```python
from build123d import *

# Parameters (mm, degrees)
BOSS_EXTRUDE1_DEPTH = 546.1
SKETCH2_R           = 49.5046
SKETCH2_R_2         = 47.6885
BOSS_EXTRUDE2_DEPTH = 203.2
BOSS_EXTRUDE3_START = 101.6
SKETCH3_R           = 49.5046
SKETCH3_R_2         = 47.6885
BOSS_EXTRUDE3_DEPTH = 101.6
SKETCH4_R           = 3.175
CUT_EXTRUDE1_DEPTH  = 753.563552693
CIRPATTERN1_COUNT   = 4


with BuildPart() as part:
    # Sketch1 → Boss-Extrude1 (new body)
    with BuildSketch(Plane.XY):
        with BuildLine():
            Line((-49.5046, 0), (-47.6885, 0))
            ThreePointArc((-47.6885, 0), (0, -47.6885), (47.6885, 0))
            Line((47.6885, 0), (49.5046, 0))
            ThreePointArc((49.5046, 0), (0, -49.5046), (-49.5046, 0))
        make_face()
    extrude(amount=BOSS_EXTRUDE1_DEPTH)

    # Sketch2 → Boss-Extrude2 (add)
    with BuildSketch(Plane.XY.offset(546.1)):
        Circle(SKETCH2_R)
        Circle(SKETCH2_R_2, mode=Mode.SUBTRACT)
    extrude(amount=BOSS_EXTRUDE2_DEPTH)

    # Sketch3 → Boss-Extrude3 (add)
    with BuildSketch(Plane(origin=(0, 0, 0), x_dir=(-1, 0, 0), z_dir=(0, 0, -1)).offset(BOSS_EXTRUDE3_START)):
        Circle(SKETCH3_R)
        Circle(SKETCH3_R_2, mode=Mode.SUBTRACT)
    extrude(amount=-BOSS_EXTRUDE3_DEPTH)

    # Sketch4 → Cut-Extrude1 (cut, through all)
    with BuildSketch(Plane(origin=(0, 0, 0), x_dir=(1, 0, 0), z_dir=(0, 1, 0))):
        with Locations(Location((0, -698.5, 0), (0, 0, 270))):
            Circle(SKETCH4_R)
    cut_extrude1 = extrude(amount=-CUT_EXTRUDE1_DEPTH, mode=Mode.SUBTRACT)

    # CirPattern1: Cut-Extrude1 ×4 about axis
    cirpattern1_axis = Axis((0, 0, 546.1), (0, 0, -1))
    for i in range(1, CIRPATTERN1_COUNT):
        add(cut_extrude1.rotate(cirpattern1_axis, i * 360 / CIRPATTERN1_COUNT), mode=Mode.SUBTRACT)


solid = part.part
```
Model file for the job. Use its own axes, mm. Coordinates: 2 decimals unless noted, no trailing zeros. Order: outer loops, then holes, each group sorted by start corner. A loop starts at its lowest first (then second) coordinate and runs counter-clockwise, first axis right, second up. Notation, with made-up numbers: (-38.5, 57.5) - (12.5, 57.5) arc R14 ccw to (12.5, 80.5) - close; hole circle Ø11 at (62.5, 39). An arc over 180 degrees is marked (long way). Return JSON: item names as keys, results as strings. Group by question number.
1) Saw through at C-C, the plane y = 26. Write the cut outline in (x, z).
2) Saw through at B-B, the plane y = -36.5. Write the cut outline in (x, z), plus the area to 3 significant figures.
3) Saw through at A-A, the plane x = 40. Write the cut outline in (y, z), plus the area to 3 significant figures.
4) Probe line 1 (Y direction, x = -3, z = 511); line 2 (Z direction, x = 0, y = -48.2) (3 decimals); line 3 (X direction, y = -24, z = 492). List the from-to ranges inside material, lowest first. Write a range as from..to.
5) Mould opens along Z. For faces 1 (the flat face through (26, 41, -101.6)), 2 (the flat face through (0, 49, 546.1)), 3 (the flat face through (-26, 41, 749.3)) say: released by +Z, released by -Z, zero draft, split by the parting line, or undercut.
6) Flat gauge pins, fed straight in: P1, Ø12, axis at x = 14.5, z = 80, coming from the +Y side; P2, Ø1.5, axis at y = -16.5, z = 483, coming from the -X side; P3, Ø6, axis at x = -8, z = 636, coming from the +Y side; P4, Ø25, axis at x = -18, y = 16.5, coming from the +Z side. Where does each tip first touch, or does it go through?
7) Saw through at D-D, the plane z = 184. Write the cut outline in (x, y), plus the area to 3 significant figures.
Values found:
{
 "1": {"outline": "(-42.13, -101.6) - (-39.98, -101.6) - (-39.98, 0) - (-42.13, 0) - close; (-42.13, 546.1) - (-39.98, 546.1) - (-39.98, 749.3) - (-42.13, 749.3) - close; (39.98, -101.6) - (42.13, -101.6) - (42.13, 0) - (39.98, 0) - close; (39.98, 546.1) - (42.13, 546.1) - (42.13, 749.3) - (39.98, 749.3) - close"},
 "2": {"outline": "(-33.44, -101.6) - (-30.69, -101.6) - (-30.69, 749.3) - (-33.44, 749.3) - close; (30.69, -101.6) - (33.44, -101.6) - (33.44, 749.3) - (30.69, 749.3) - close", "area": "4,680 mm²"},
 "3": {"outline": "(-29.17, -101.6) - (-25.97, -101.6) - (-25.97, 749.3) - (-29.17, 749.3) - close; (25.97, -101.6) - (29.17, -101.6) - (29.17, 0) - (25.97, 0) - close; (25.97, 546.1) - (29.17, 546.1) - (29.17, 749.3) - (25.97, 749.3) - close", "area": "3,700 mm²"},
 "4": {"line 1": "y = -49.41..-47.59", "line 2": "z = -101.6..695.325, 701.675..749.3", "line 3": "x = -43.3..-41.21, 41.21..43.3"},
 "5": {"face 1": "released by -Z", "face 2": "undercut", "face 3": "released by +Z"},
 "6": {"P1": "stops at y = -43.06", "P2": "stops at x = -46.93", "P3": "stops at y = 49.25", "P4": "passes through"},
 "7": {"outline": "(-49.5, 0) arc R49.5 ccw to (49.5, 0) - (47.69, 0) arc R47.69 cw to (-47.69, 0) - close", "area": "277 mm²"}
}
